from build123d import *

# Parameters (mm, degrees)
SKETCH1_R         = 75.819
EXTRUDE1_DEPTH    = 19.812
SKETCH2_R         = 4.2164
EXTRUDE2_DEPTH    = 19.812
CIRPATTERN1_COUNT = 16
SKETCH3_R         = 22.225
SKETCH3_R_2       = 20.574
EXTRUDE3_DEPTH    = 127
EXTRUDE4_REACH    = 168.211
SKETCH4_R         = 20.574
SKETCH6_R         = 34.671
SKETCH6_R_2       = 20.574
EXTRUDE5_DEPTH    = 12.7
EXTRUDE6_REACH    = 183.799
SKETCH7_R         = 3.3655
CIRPATTERN2_COUNT = 6
SKETCH10_R        = 9.525
SKETCH10_R_2      = 8.636
EXTRUDE7_DEPTH    = 330.2
EXTRUDE8_REACH    = 404.651
SKETCH10_2_R      = 9.525
SKETCH10_2_R_2    = 8.636
SKETCH11_R        = 8.636
EXTRUDE9_DEPTH    = 403.65117179
CIRPATTERN3_COUNT = 6


with BuildPart() as part:
    # Sketch1 → Extrude1 (new body)
    with BuildSketch(Plane(origin=(0, 0, 0), x_dir=(1, 0, 0), z_dir=(0, 1, 0))):
        with Locations(Location((0, 0, 0), (0, 0, 270))):
            Circle(SKETCH1_R)
    extrude(amount=EXTRUDE1_DEPTH)

    # Sketch2 → Extrude2 (cut)
    with BuildSketch(Plane(origin=(0, 19.812, 0), x_dir=(1, 0, 0), z_dir=(0, 1, 0))):
        with Locations(Location((0, 65.1256, 0), (0, 0, 270))):
            Circle(SKETCH2_R)
    extrude2 = extrude(amount=-EXTRUDE2_DEPTH, mode=Mode.SUBTRACT)

    # CirPattern1: Extrude2 ×16 about axis
    cirpattern1_axis = Axis((0, 0, 0), (0, 1, 0))
    for i in range(1, CIRPATTERN1_COUNT):
        add(extrude2.rotate(cirpattern1_axis, i * 360 / CIRPATTERN1_COUNT), mode=Mode.SUBTRACT)

    # Sketch3 → Extrude3 (add)
    with BuildSketch(Plane(origin=(0, 19.812, 0), x_dir=(1, 0, 0), z_dir=(0, 1, 0))):
        with Locations(Location((0, 0, 0), (0, 0, 270))):
            Circle(SKETCH3_R)
        with Locations(Location((0, 0, 0), (0, 0, 270))):
            Circle(SKETCH3_R_2, mode=Mode.SUBTRACT)
    extrude(amount=EXTRUDE3_DEPTH)

    # Sketch4 → Extrude4 (cut, up to next)
    with BuildSketch(Plane(origin=(0, 19.812, 0), x_dir=(1, 0, 0), z_dir=(0, 1, 0)), mode=Mode.PRIVATE) as extrude4_sk1:
        with Locations(Location((0, 0, 0), (0, 0, 270))):
            Circle(SKETCH4_R)
    extrude4_tool1 = extrude(extrude4_sk1.sketch, amount=-EXTRUDE4_REACH, mode=Mode.PRIVATE) & part.part
    add(extrude4_tool1.solids().sort_by_distance((0, 19.812, 0))[0], mode=Mode.SUBTRACT)

    # Sketch6 → Extrude5 (add)
    with BuildSketch(Plane(origin=(0, 146.812, 0), x_dir=(1, 0, 0), z_dir=(0, 1, 0))):
        with Locations(Location((0, 0, 0), (0, 0, 270))):
            Circle(SKETCH6_R)
        with Locations(Location((0, 0, 0), (0, 0, 270))):
            Circle(SKETCH6_R_2, mode=Mode.SUBTRACT)
    extrude(amount=-EXTRUDE5_DEPTH)

    # Sketch7 → Extrude6 (cut, up to next)
    with BuildSketch(Plane(origin=(0, 146.812, 0), x_dir=(1, 0, 0), z_dir=(0, 1, 0)), mode=Mode.PRIVATE) as extrude6_sk1:
        with Locations(Location((0, 29.3624, 0), (0, 0, 270))):
            Circle(SKETCH7_R)
    extrude6_tool1 = extrude(extrude6_sk1.sketch, amount=-EXTRUDE6_REACH, mode=Mode.PRIVATE) & part.part
    extrude6 = extrude6_tool1.solids().sort_by_distance((0, 146.812, -29.3624))[0]
    add(extrude6, mode=Mode.SUBTRACT)

    # CirPattern2: Extrude6 ×6 about axis
    cirpattern2_axis = Axis((0, 0, 0), (0, 1, 0))
    for i in range(1, CIRPATTERN2_COUNT):
        add(extrude6.rotate(cirpattern2_axis, i * 360 / CIRPATTERN2_COUNT), mode=Mode.SUBTRACT)

    # Sketch10 → Extrude7 (add)
    with BuildSketch(Plane(origin=(0, -241.3, 0), x_dir=(-1, 0, 0), z_dir=(0, 0.992546151641322, 0.12186934340514811))):
        with Locations(Location((0, 0, 0), (0, 0, 253.960195481))):
            Circle(SKETCH10_R)
        with Locations(Location((0, 0, 0), (0, 0, 270))):
            Circle(SKETCH10_R_2, mode=Mode.SUBTRACT)
    extrude7 = extrude(amount=EXTRUDE7_DEPTH)

    # Extrude8: up to this face of the body (flat: up to its plane)
    extrude8_end = Plane(part.part.faces().sort_by_distance((0, 0, -73.674514838))[0])
    # Sketch10<2> → Extrude8 (cut, up to the picked face)
    with BuildSketch(Plane(origin=(0, -241.3, 0), x_dir=(-1, 0, 0), z_dir=(0, 0.992546151641322, 0.12186934340514811)), mode=Mode.PRIVATE) as extrude8_sk1:
        with Locations(Location((0, 0, 0), (0, 0, 270))):
            Circle(SKETCH10_2_R)
        with Locations(Location((0, 0, 0), (0, 0, 270))):
            Circle(SKETCH10_2_R_2, mode=Mode.SUBTRACT)
    extrude8_tool1 = split(extrude(extrude8_sk1.sketch, amount=EXTRUDE8_REACH, mode=Mode.PRIVATE), bisect_by=extrude8_end, keep=Keep.BOTH, mode=Mode.PRIVATE)
    extrude8 = extrude8_tool1.solids().sort_by(Axis((0, -242.427973, 9.186603), (0, 0.992546151641322, 0.12186934340514811)))[0]
    add(extrude8, mode=Mode.SUBTRACT)

    # Sketch11 → Extrude9 (cut, through all)
    with BuildSketch(Plane(origin=(0, -241.3, 0), x_dir=(-1, 0, 0), z_dir=(0, 0.992546151641322, 0.12186934340514811))):
        with Locations(Location((0, 0, 0), (0, 0, 270))):
            Circle(SKETCH11_R)
    extrude9 = extrude(amount=EXTRUDE9_DEPTH, mode=Mode.SUBTRACT)

    # CirPattern3: Extrude7, Extrude8, Extrude9 ×6 about axis
    cirpattern3_axis = Axis((0, 0, 0), (0, 1, 0))
    add([extrude7.rotate(cirpattern3_axis, i * 360 / CIRPATTERN3_COUNT) for i in range(1, CIRPATTERN3_COUNT)])
    add([extrude8.rotate(cirpattern3_axis, i * 360 / CIRPATTERN3_COUNT) for i in range(1, CIRPATTERN3_COUNT)], mode=Mode.SUBTRACT)
    add([extrude9.rotate(cirpattern3_axis, i * 360 / CIRPATTERN3_COUNT) for i in range(1, CIRPATTERN3_COUNT)], mode=Mode.SUBTRACT)


solid = part.part
Verification items for the finished model (mm, model axes). A direction names the side the tool comes from. Give positions to 0.01 mm unless a question says otherwise; leave off trailing zeros. Loops run counter-clockwise (first coordinate to the right, second up) from the corner with the lowest first, then second, coordinate; pieces in that order, holes last.
1) Sectioned sample at B-B, the plane y = 98. Enter the section's corners in (x, z) (3 decimals), then the cut area to 3 significant figures.
2) Set-up check for faces 1 (the flat face through (-43.33, 85.68, -17.82)), 2 (the flat face through (-37.099, 85.678, 28.618)), 3 (the cylindrical face through (-24.42, 140.55, 17.89)), 4 (the flat face through (-23, 134.112, 0)), 5 (the flat face through (43.33, 85.68, 17.82)): record each of +Z, -Z, +X, -X, +Y, -Y from which the full face is reachable in a straight line by a thin tool's end or side.
3) Sectioned sample at C-C, the plane y = 11.5. Count the separate pieces of the cut face and the enclosed holes in it, then the cut area to 3 significant figures.
4) Draft check along Y on faces 6 (the cylindrical face through (17.51, 1.69, -10.15)), 7 (the cylindrical face through (30.539, 42.566, 8.785)), 8 (the cylindrical face through (26.706, 10.045, -63.989)). Enter one of: pulls with the +Y half, pulls with the -Y half, needs draft (parallel to the pull), parting line crosses it, or undercut.
5) Thickness scan on line 1 along Y through (x, z) = (-33, 7.5); line 2 along Z through (x, y) = (34.5, 35.5); line 3 along X through (y, z) = (62.5, 36.5). Record the ranges inside material, lowest first.
6) Depth check by flat-ended pin: pin 1 Ø6 at (x, z) = (0, 29.36) entering from +Y; pin 2 Ø4 at (x, y) = (-33, 67) entering from -Z; pin 3 Ø4 at (x, y) = (-3.5, 42) entering from +Z. Enter the tip coordinate at first touch or a pass-through.
7) Sectioned sample at A-A, the plane z = 0. Enter the section's corners in (x, y) (3 decimals).
Answers:
1. outline: circle Ø44.45 at (0, 0); hole circle Ø41.148 at (0, 0)
1. area: 222 mm2
2. face 1: -Z, -X
2. face 2: +Z, -X
2. face 3: +Y
2. face 4: none
2. face 5: +Z, +X
3. separate pieces: 1
3. enclosed holes: 23
3. area: 14,400 mm2
4. face 6: pulls with the +Y half
4. face 7: undercut
4. face 8: needs draft
5. line 1: y = 0 to 19.81, 134.11 to 146.81
5. line 2: z = -25.12 to -24.05, -10 to -8.93, 8.93 to 10, 24.05 to 25.12
5. line 3: x = -9.49 to -8.6, 8.6 to 9.49
6. pin 1: stops at y = 87.6
6. pin 2: stops at z = -28.59
6. pin 3: stops at z = 44.34
7. outline: (-75.819, 0) - (-69.342, 0) - (-69.342, 19.812) - (-75.819, 19.812) - close; (-60.909, 0) - (-20.574, 0) - (-20.574, 146.812) - (-34.671, 146.812) - (-34.671, 134.112) - (-22.225, 134.112) - (-22.225, 19.812) - (-60.909, 19.812) - close; (20.574, 0) - (60.909, 0) - (60.909, 19.812) - (22.225, 19.812) - (22.225, 134.112) - (34.671, 134.112) - (34.671, 146.812) - (20.574, 146.812) - close; (69.342, 0) - (75.819, 0) - (75.819, 19.812) - (69.342, 19.812) - close
